Geometry check sheet. Reference: drawing and pictorial views, mm from the part's lowest x, y, z. A direction names the side the tool comes from. Coordinates: 2 decimals unless noted, no trailing zeros. Loops run counter-clockwise (first coordinate to the right, second up) from the corner with the lowest first, then second, coordinate; pieces in that order, holes last. Notation, with made-up numbers: (-26, 18) -> (0, 18) arc R33 ccw to (0, 53) -> close; hole circle Ø7 at (-31.75, 25). An arc over 180 degrees is marked (long way). Answer as a JSON object with one key per item and string values.
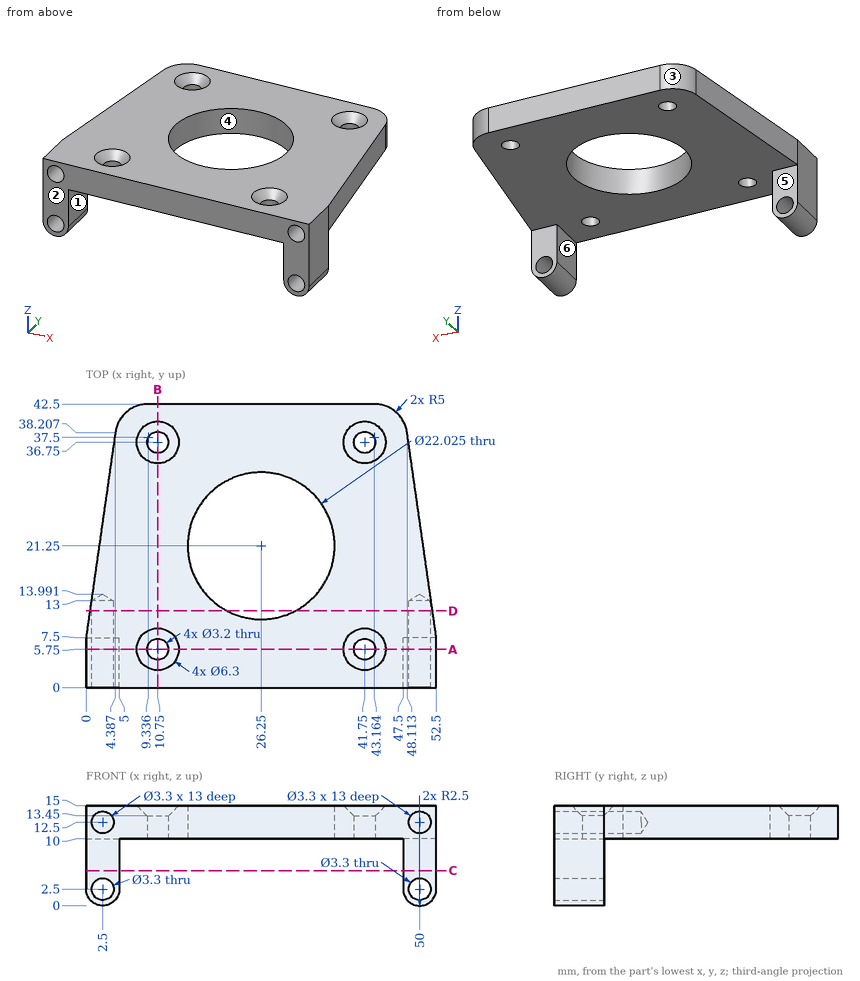
1. Mould release check, pull along X, two halves, no side actions. Record for the marked faces 1, 2 and 3: released by +X, released by -X, zero draft, split by the parting line, or undercut.
Evaluation:
{"face 1": "undercut", "face 2": "zero draft", "face 3": "released by -X"}
2. Depth check by flat-ended pin: P1, Ø5.5, axis at x = 49.5, z = 5, coming from the +Y side; P2, Ø1.5, axis at y = 22, z = 12.5, coming from the +X side; P3, Ø5, axis at y = 38, z = 11.5, coming from the +X side. Enter the tip coordinate at first touch or a pass-through.
Evaluation:
{"P1": "stops at y = 7.5", "P2": "stops at x = 50.54", "P3": "stops at x = 48.5"}
3. Section check C-C, the plane z = 5.25. Record the boundary of the cut face in (x, y), then the cut area to 3 significant figures.
Evaluation:
{"outline": "(0, 0) -> (5, 0) -> (5, 7.5) -> (0, 7.5) -> close; (47.5, 0) -> (52.5, 0) -> (52.5, 7.5) -> (47.5, 7.5) -> close", "area": "75.0 mm^2"}
4. Section check A-A, the plane y = 5.75. Record the boundary of the cut face in (x, z).
Evaluation:
{"outline": "(0, 2.5) arc R2.5 ccw to (5, 2.5) -> (5, 10) -> (9.15, 10) -> (9.15, 13.45) -> (7.6, 15) -> (0, 15) -> close; (12.35, 10) -> (40.15, 10) -> (40.15, 13.45) -> (38.6, 15) -> (13.9, 15) -> (12.35, 13.45) -> close; (43.35, 10) -> (47.5, 10) -> (47.5, 2.5) arc R2.5 ccw to (52.5, 2.5) -> (52.5, 15) -> (44.9, 15) -> (43.35, 13.45) -> close; hole circle Ø3.3 at (2.5, 2.5); hole circle Ø3.3 at (2.5, 12.5); hole circle Ø3.3 at (50, 2.5); hole circle Ø3.3 at (50, 12.5)"}
5. Section check B-B, the plane x = 10.75. Record the boundary of the cut face in (y, z).
Evaluation:
{"outline": "(0, 10) -> (4.15, 10) -> (4.15, 13.45) -> (2.6, 15) -> (0, 15) -> close; (7.35, 10) -> (35.15, 10) -> (35.15, 13.45) -> (33.6, 15) -> (8.9, 15) -> (7.35, 13.45) -> close; (38.35, 10) -> (42.5, 10) -> (42.5, 15) -> (39.9, 15) -> (38.35, 13.45) -> close"}
6. Tool access check on the marked faces 4, 5 and 6. Record the directions out of +Z, -Z, +X, -X, +Y, -Y that give a thin tool (end or side, any length) a straight path to the whole face; none if there is none.
Evaluation:
{"face 4": "+Z, -Z", "face 5": "-Z, +X, -X, +Y", "face 6": "-Z, +Y, -Y"}
7. Thickness scan on probe 1 along X at (y, z) = (6.25, 2.5); probe 2 along Y at (x, z) = (10.75, 12.3); probe 3 along Z at (x, y) = (50, 4.75). Record the ranges inside material, lowest first. Write a range as from..to.
Evaluation:
{"probe 1": "x = 0..0.85, 4.15..5, 47.5..48.35, 51.65..52.5", "probe 2": "y = 0..4.15, 7.35..35.15, 38.35..42.5", "probe 3": "z = 0..0.85, 4.15..10.85, 14.15..15"}
8. Section check D-D, the plane y = 11.5. Record the boundary of the cut face in (x, z).
Evaluation:
{"outline": "(0.57, 10) -> (21.13, 10) -> (21.13, 15) -> (0.57, 15) -> close; (31.37, 10) -> (51.93, 10) -> (51.93, 15) -> (31.37, 15) -> close; hole circle Ø3.3 at (2.5, 12.5); hole circle Ø3.3 at (50, 12.5)"}
